Autodesk Inventor part; units mm, degrees
ref_plane "YZ Plane" through (0, 0, 0) normal (1, 0, 0) x (0, 1, 0)
ref_plane "XZ Plane" through (0, 0, 0) normal (0, 1, 0) x (-1, 0, 0)
ref_plane "XY Plane" through (0, 0, 0) normal (0, 0, 1) x (1, 0, 0)
sketch "Sketch1" plane through (0, 0, 0) normal (0, 0, 1) x (1, 0, 0)
  line L0 (12.7, 0) -> (12.7, 24.13)
  line L1 (0, 24.13) -> (0, 0)
  line L2 (3.81, 24.13) -> (8.89, 24.13)
  line L3 (8.89, 24.13) -> (8.89, 26.924)
  line L4 (8.89, 26.924) -> (3.81, 26.924)
  line L5 (3.81, 26.924) -> (3.81, 24.13)
  line L6 (3.81, 0) -> (8.89, 0)
  line L7 (8.89, 0) -> (8.89, -2.794)
  line L8 (8.89, -2.794) -> (3.81, -2.794)
  line L9 (3.81, -2.794) -> (3.81, 0)
  line L10 (12.7, 24.13) -> (8.89, 24.13)
  line L11 (3.81, 24.13) -> (0, 24.13)
  line L12 (0, 0) -> (3.81, 0)
  line L13 (8.89, 0) -> (12.7, 0)
  line L14 (-1.7824, 25.8737) -> (3.334, 25.8737)
  line L15 (3.334, 25.8737) -> (3.334, 28.6416)
  line L16 (3.334, 28.6416) -> (9.4568, 28.6416)
  line L17 (9.4568, 28.6416) -> (9.4568, 25.8737)
  line L18 (9.4568, 25.8737) -> (14.3215, 25.8737)
  dimension "d0" = 12.7
  dimension "d1" = 24.13
  dimension "d2" = 5.08
  dimension "d3" = 2.794
  dimension "d4" = 3.81
  dimension "d5" = 5.08
  dimension "d6" = 2.794
  dimension "d7" = 3.81
extrude "Extrusion1" add sketch "Sketch1" along normal blind 82.55
sketch "Sketch2" plane through (12.7, 0, 0) normal (1, 0, 0) x (0, 0, -1)
  line L0 (-82.55, 24.13) -> (-82.55, 0)
  circle A0 centre (-82.55, 12.065) radius 13.335
  point P0 (0, 0)
  dimension "d10" = 26.67
extrude "Extrusion2" cut sketch "Sketch2" against normal blind 82.55
properties part number "EngineClip"
Part model, mm, in its own coordinate system. A direction names the side the tool comes from. Round coordinates to 2 decimals unless told otherwise and drop trailing zeros. Write each loop counter-clockwise with the first axis right and the second up, starting at its lowest first coordinate (ties: lowest second). Pieces come first, ordered by that corner, then holes. Notation, with made-up numbers: M 43,-38.5 L 78,-38.5 A28 cw 78,-2.5 Z; hole C 65.25,42.5 d3. An arc over 180 degrees is marked long. Return JSON: item names as keys, results as strings. Group by question number.
(1) Saw through at D-D on x = 11. Write the cut outline in (y, z) (3 decimals), then the cut area to 3 significant figures.
(2) Two-plate mould, pull along Y, no slides. Class faces 6 (the face through (6.44, 11.77, 69.22)), 7 (the face through (11, 0, 38)), 8 (the face through (8.89, -1, 41)): +Y half, -Y half, draft (parallel to the pull), parting line (faces both ways), or undercut.
(3) Pin check, flat tips, straight feed: pin 1 Ø4 at (x, z) = (11.5, 33) entering from -Y; pin 2 Ø0.8 at (y, z) = (26, 30) entering from +X; pin 3 Ø1 at (x, y) = (10, 5.5) entering from +Z. Stop position of each tip, or through.
(4) Saw through at B-B on z = 47.5. Write the cut outline in (x, y).
(5) Saw through at C-C on y = 5.25. Write the cut outline in (x, z).
(6) Drill centre lines: probe 1 along Y at (x, z) = (11.5, 49); probe 2 along Y at (x, z) = (4.5, 71); probe 3 along Z at (x, y) = (3.5, 12.5). Where is each one in solid material? Low to high.
(7) Saw through at A-A on x = 4.75. Write the cut outline in (y, z) (3 decimals), then the cut area to 3 significant figures.
(8) Which spindle directions (+Z, -Z, +X, -X, +Y, -Y) get a long thin tool onto all of the face, cutting with end or side? Do faces 1 (the face through (3.81, -1, 41)), 2 (the face through (11, 24.13, 38)), 3 (the face through (0, 12, 38)), 4 (the face through (3.81, 26, 41)), 5 (the face through (6, -2, 82.55)). Say none if no direction does.
Returned:
{
 "1": {"outline": "M 0,0 L 24.13,0 L 24.13,76.87 A13.335 cw 0,76.87 Z", "area": "1,720 mm²"},
 "2": {"face 6": "undercut", "face 7": "-Y half", "face 8": "draft"},
 "3": {"pin 1": "y = 0", "pin 2": "x = 8.89", "pin 3": "z = 71.24"},
 "4": {"outline": "M 0,0 L 3.81,0 L 3.81,-2.79 L 8.89,-2.79 L 8.89,0 L 12.7,0 L 12.7,24.13 L 8.89,24.13 L 8.89,26.92 L 3.81,26.92 L 3.81,24.13 L 0,24.13 Z"},
 "5": {"outline": "M 0,0 L 12.7,0 L 12.7,71.09 L 0,71.09 Z"},
 "6": {"probe 1": "0 to 24.13", "probe 2": "-2.79 to 5.4, 18.73 to 26.92", "probe 3": "0 to 69.22"},
 "7": {"outline": "M -2.794,0 L 26.924,0 L 26.924,82.55 L 25.4,82.55 A13.335 cw -1.27,82.55 L -2.794,82.55 Z", "area": "2,170 mm²"},
 "8": {"face 1": "+Z, -Z, -X, -Y", "face 2": "+Z, -Z, +X, +Y", "face 3": "+Z, -Z, -X, +Y, -Y", "face 4": "+Z, -Z, -X, +Y", "face 5": "+Z, +X, -X, +Y, -Y"}
}
